The listing builds one solid part. Answer for the finished solid, in the listing's coordinates (mm). A direction names the side the tool comes from. Give positions to 0.01 mm unless a question says otherwise; leave off trailing zeros. Loops run counter-clockwise (first coordinate to the right, second up) from the corner with the lowest first, then second, coordinate; pieces in that order, holes last. Notation, with made-up numbers: (-6, 43.25) - (32, 43.25) arc R16 cw to (32, 71.25) - close; hole circle Ø1 at (78, 55). An arc over 180 degrees is marked (long way). Answer in a Markdown table with one row per item. Add a question column.
```python
from build123d import *

# Parameters (mm, degrees)
SKETCH1_W         = 24
SKETCH1_H         = 24.5
SKETCH1_W_2       = 39
SKETCH1_H_2       = 19
CHAMFER9_SIZE     = 6
CHAMFER9_SIZE2    = 4
HOLE1_D           = 13
HOLE1_DEPTH       = 16
HOLE1_CBORE_D     = 28
HOLE1_CBORE_DEPTH = 7.5


with BuildPart() as part:
    # Sketch1 → Revolve2 (revolve)
    with BuildSketch(Plane(origin=(0, 0, 0), x_dir=(0, 0, -1), z_dir=(1, 0, 0)), mode=Mode.PRIVATE) as revolve2_sk:
        with Locations((12, 12.25)):
            Rectangle(SKETCH1_W, SKETCH1_H)
        Polygon((24, 19.25), (24, 0), (30, 0), (30, 19), (30, 19.25), align=None)
        with Locations((49.5, 9.5)):
            Rectangle(SKETCH1_W_2, SKETCH1_H_2)
    revolve(revolve2_sk.sketch.rotate(Axis((0, 0, 0), (0, 0, -1)), 90), axis=Axis((0, 0, 0), (0, 0, -1)))

    # Chamfer9
    chamfer9_edges = [part.edges().sort_by_distance(p)[0] for p in [
        (-19, 0, -69),
    ]]
    chamfer9_side = [part.faces().sort_by_distance(p)[0] for p in [
        (0, 0, -69),
    ]]
    chamfer(chamfer9_edges, length=CHAMFER9_SIZE, length2=CHAMFER9_SIZE2, reference=chamfer9_side[0])

    # Cut-Loft1: read off the stored shape, not the designer's step
    # Cut-Loft1: loft between two sections, ruled curve by curve
    cut_loft1_from = [
        Edge.make_bspline([(14.330823066, 14.658700837, 0), (43.648224741, -14.002945296, 0), (14.986578608, -43.32034697, 0), (-14.330823066, -14.658700837, 0), (-43.648224741, 14.002945296, 0), (-14.986578608, 43.32034697, 0), (14.330823066, 14.658700837, 0)], [0, 0, 0, 0, 0.5, 0.5, 0.5, 1, 1, 1, 1], 3, [1, 0.333333333, 0.333333333, 1, 0.333333333, 0.333333333, 1]),
    ]
    cut_loft1_to = [
        Edge.make_bspline([(13.812637818, 8.07533507, -12), (29.963307959, -19.549940567, -12), (2.338032322, -35.700610707, -12), (-13.812637818, -8.07533507, -12), (-29.963307959, 19.549940567, -12), (-2.338032322, 35.700610707, -12), (13.812637818, 8.07533507, -12)], [0, 0, 0, 0, 0.5, 0.5, 0.5, 1, 1, 1, 1], 3, [1, 0.333333333, 0.333333333, 1, 0.333333333, 0.333333333, 1]),
    ]
    cut_loft1 = Solid(Shell([*[Face.make_surface_from_curves(cut_loft1_from[k], cut_loft1_to[k]) for k in range(1)], Face(Wire(cut_loft1_from)), Face(Wire(cut_loft1_to))]))
    add(cut_loft1, mode=Mode.SUBTRACT)

    # Hole1
    with Locations(Plane.XY.offset(-12)):
        with Locations((0, 0)):
            CounterBoreHole(HOLE1_D / 2, HOLE1_CBORE_D / 2, HOLE1_CBORE_DEPTH, depth=HOLE1_DEPTH)


solid = part.part
```
(1) A cutting plane is placed at B-B on z = -51. Determine the outline of the cut face in (x, y).
(2) A tool of negligible diameter and unlimited length cuts with its end or side. For faces 4 (the face through (13.5, -5.1, -12)), 5 (the face through (-4.119, 18.548, -47.745)), 6 (the face through (0, 0, -69)), from which of +Z, -Z, +X, -X, +Y, -Y can it reach the whole face along a straight path? Write none if from no direction.
(3) Given pin 1 Ø1 at (x, z) = (-18, -33.5) entering from -Y; pin 2 Ø5 at (x, y) = (-14, -16) entering from -Z; pin 3 Ø11.5 at (x, y) = (0, 0) entering from +Z, each flat-ended and moving along its own axis, determine where each tip first touches the part or whether it passes through.
(4) Find the intervals of material crossed by line 1 along Y through (x, z) = (0, -23.75); line 2 along Y through (x, z) = (0, -17); line 3 along Z through (x, y) = (7.5, 22.5), in increasing order. Write a range as [from, to].
(5) The mould has two halves that part along Y. Classify faces 1 (the face through (3, -6, -19.5)), 2 (the face through (20, -7, 0)), 3 (the face through (-15.28, 11.71, -26.96)): pulls with the +Y half, pulls with the -Y half, needs draft (parallel to the pull), parting line crosses it, or undercut.
(6) A cutting plane is placed at A-A on z = -25. Determine the outline of the cut face in (x, y).
Evaluation:
| question | item | result |
|---|---|---|
| 1 | outline | circle Ø38 at (0, 0) |
| 2 | face 4 | +Z |
| 2 | face 5 | -Z |
| 2 | face 6 | -Z, +X, -X, +Y, -Y |
| 3 | pin 1 | stops at y = -7.4 |
| 3 | pin 2 | stops at z = -65.16 |
| 3 | pin 3 | stops at z = -28 |
| 4 | line 1 | y = [-24.5, -6.5], [6.5, 24.5] |
| 4 | line 2 | y = [-24.5, -14], [14, 24.5] |
| 4 | line 3 | z = [-24, 0] |
| 5 | face 1 | undercut |
| 5 | face 2 | needs draft |
| 5 | face 3 | parting line crosses it |
| 6 | outline | circle Ø38.5 at (0, 0); hole circle Ø13 at (0, 0) |
